Read the model definition and answer for the solid it produces. Units are mm, in the model's axes. A direction names the side the tool comes from. Coordinates: 2 decimals unless noted, no trailing zeros. Write each loop counter-clockwise with the first axis right and the second up, starting at its lowest first coordinate (ties: lowest second). Pieces come first, ordered by that corner, then holes.
(1) Section B-B on x = 16.5 is taken. Write down the section's boundary in (y, z) (1 decimal), then the cut area to 3 significant figures.
(2) Which of the six approach directions +Z, -Z, +X, -X, +Y, -Y give full straight-line access (tool end or side, diameter ignored) to faces 1 (the cylindrical face through (4.7, 9.72, -16.59)), 2 (the flat face through (9.525, 9, -9))?
(3) The mould has two halves that part along Y. Classify faces 3 (the flat face through (9, 0, -38)), 4 (the flat face through (9, 19, -76.2)), 5 (the flat face through (10, 38.1, -64)), 6 (the flat face through (9.525, 9, -60)): +Y half, -Y half, draft (parallel to the pull), parting line (faces both ways), or undercut.
(4) Find the intervals of material crossed by probe 1 along Y at (x, z) = (4.75, -12.7); probe 2 along Y at (x, z) = (15.25, -12.5); probe 3 along Z at (x, y) = (3.5, 15), in increasing order.
(5) Section A-A on y = 12.7 is taken. State how many separate pieces and enclosed holes the cut face has, then the cut area to 3 significant figures.
(6) Given pin 1 (6 mm diameter, centred on x = 8.5, z = -39.5, fed in from +Y), flat-ended and moving along its own axis, determine where the tip first touches the part or whether it passes through.
(7) Section D-D on y = 32 is taken. Write down the section's boundary in (x, z), then the cut area to 3 significant figures.
from build123d import *

# Parameters (mm, degrees)
SKETCH1_W                                        = 76.2
SKETCH1_H                                        = 76.2
BOSS_EXTRUDE1_DEPTH                              = 19.05
SKETCH2_R                                        = 13.096875
CUT_EXTRUDE1_DEPTH                               = 110.433918417
CBORE_FOR_3_8_SOCKET_HEAD_CAP_SCREW1_D           = 9.8044
CBORE_FOR_3_8_SOCKET_HEAD_CAP_SCREW1_CBORE_D     = 15.875
CBORE_FOR_3_8_SOCKET_HEAD_CAP_SCREW1_CBORE_DEPTH = 9.525
SKETCH5_W                                        = 76.2
SKETCH5_H                                        = 38.1
CUT_EXTRUDE2_DEPTH                               = 110.433918417


with BuildPart() as part:
    # Sketch1 → Boss-Extrude1 (new body)
    with BuildSketch(Plane(origin=(0, 0, 0), x_dir=(0, 0, -1), z_dir=(1, 0, 0))):
        with Locations((38.1, 38.1)):
            Rectangle(SKETCH1_W, SKETCH1_H)
    extrude(amount=BOSS_EXTRUDE1_DEPTH)

    # Sketch2 → Cut-Extrude1 (cut, through all)
    with BuildSketch(Plane(origin=(19.05, 0, 0), x_dir=(0, 0, -1), z_dir=(1, 0, 0))):
        with Locations((38.1, 38.1)):
            Circle(SKETCH2_R)
    extrude(amount=-CUT_EXTRUDE1_DEPTH, mode=Mode.SUBTRACT)

    # CBORE for 3/8 Socket Head Cap Screw1 (through all)
    with Locations(Plane(origin=(19.05, 0, 0), x_dir=(0, 0, -1), z_dir=(1, 0, 0))):
        with Locations((12.7, 12.7), (63.5, 12.7)):
            CounterBoreHole(CBORE_FOR_3_8_SOCKET_HEAD_CAP_SCREW1_D / 2, CBORE_FOR_3_8_SOCKET_HEAD_CAP_SCREW1_CBORE_D / 2, CBORE_FOR_3_8_SOCKET_HEAD_CAP_SCREW1_CBORE_DEPTH)

    # Sketch5 → Cut-Extrude2 (cut, through all)
    with BuildSketch(Plane(origin=(19.05, 0, 0), x_dir=(0, 0, -1), z_dir=(1, 0, 0))):
        with Locations((38.1, 57.15)):
            Rectangle(SKETCH5_W, SKETCH5_H)
    extrude(amount=-CUT_EXTRUDE2_DEPTH, mode=Mode.SUBTRACT)


solid = part.part
Response:
1. outline: (0, -76.2) - (38.1, -76.2) - (38.1, -51.2) arc R13.1 cw to (38.1, -25) - (38.1, 0) - (0, 0) - close; hole circle Ø15.9 at (12.7, -63.5); hole circle Ø15.9 at (12.7, -12.7)
1. area: 2,240 mm2
2. face 1: +X, -X
2. face 2: +X
3. face 3: -Y half
3. face 4: draft
3. face 5: +Y half
3. face 6: undercut
4. probe 1: y = 0 to 7.8, 17.6 to 38.1
4. probe 2: y = 0 to 4.77, 20.63 to 38.1
4. probe 3: z = -76.2 to -67.83, -59.17 to -17.03, -8.37 to 0
5. separate pieces: 3
5. enclosed holes: 0
5. area: 962 mm2
6. pin 1: stops at y = 25.76
7. outline: (0, -76.2) - (19.05, -76.2) - (19.05, -49.69) - (0, -49.69) - close; (0, -26.51) - (19.05, -26.51) - (19.05, 0) - (0, 0) - close
7. area: 1,010 mm2
